Could you check a few things on this model? Use its own coordinates, in mm. A direction names the side the tool comes from. Give positions to 0.01 mm unless a question says otherwise; leave off trailing zeros. Write each loop counter-clockwise with the first axis right and the second up, starting at its lowest first coordinate (ties: lowest second). Pieces come first, ordered by that corner, then holes. Notation, with made-up numbers: (39, 68.5) -> (93, 68.5) arc R12 ccw to (93, 91.5) -> close; hole circle Ø1 at (-3, 14). An arc over 180 degrees is marked (long way). Write item = value, one per line. Start each with the question number.
```python
from build123d import *

# Parameters (mm, degrees)
ESQUISSE1_W                = 48
ESQUISSE1_H                = 24
EXTRUSION1_DEPTH           = 7.5
CONG_2_R                   = 5
CONG_5_R                   = 1
CONG_6_R                   = 1
ESQUISSE4_W                = 0.5
ESQUISSE4_H                = 18.982849842
EXTRUSION2_DEPTH           = 0.5
ESQUISSE5_R                = 0.25
EXTRUSION3_DEPTH           = 0.5
CHANFREIN1_SIZE            = 1
ESQUISSE6_R                = 1.5
EXTRUSION6_DEPTH           = 0.5
EXTRUSION6_DRAFT           = -45
EXTRUSION6_PROFILE_2_DEPTH = 0.5
EXTRUSION6_PROFILE_2_DRAFT = -45
EXTRUSION6_PROFILE_3_DEPTH = 0.5
EXTRUSION6_PROFILE_3_DRAFT = -45
EXTRUSION6_PROFILE_4_DEPTH = 0.5
EXTRUSION6_PROFILE_4_DRAFT = -45
EXTRUSION6_PROFILE_5_DEPTH = 0.5
EXTRUSION6_PROFILE_5_DRAFT = -45
EXTRUSION6_PROFILE_6_DEPTH = 0.5
EXTRUSION6_PROFILE_6_DRAFT = -45
EXTRUSION6_PROFILE_7_DEPTH = 0.5
EXTRUSION6_PROFILE_7_DRAFT = -45
EXTRUSION6_PROFILE_8_DEPTH = 0.5
EXTRUSION6_PROFILE_8_DRAFT = -45
EXTRUSION6_PROFILE_9_DEPTH = 0.5
EXTRUSION6_PROFILE_9_DRAFT = -45


with BuildPart() as part:
    # Esquisse1 → Extrusion1 (new body)
    with BuildSketch(Plane(origin=(0, 0, 0), x_dir=(1, 0, 0), z_dir=(0, 1, 0))):
        with Locations((24, 12)):
            Rectangle(ESQUISSE1_W, ESQUISSE1_H)
    extrude(amount=EXTRUSION1_DEPTH)

    # Congé2
    cong_2_edges = [part.edges().sort_by_distance(p)[0] for p in [
        (0, 3.75, -24),
        (48, 3.75, -24),
        (48, 3.75, 0),
        (0, 3.75, 0),
    ]]
    fillet(cong_2_edges, radius=CONG_2_R)

    # Congé5
    cong_5_edges = [part.edges().sort_by_distance(p)[0] for p in [
        (48, 7.5, -12),
        (24, 7.5, 0),
        (0, 7.5, -12),
        (24, 7.5, -24),
        (1.464466094, 7.5, -22.535533906),
        (1.464466094, 7.5, -1.464466094),
        (46.535533906, 7.5, -22.535533906),
        (46.535533906, 7.5, -1.464466094),
    ]]
    fillet(cong_5_edges, radius=CONG_5_R)

    # Congé6
    cong_6_edges = [part.edges().sort_by_distance(p)[0] for p in [
        (48, 0, -12),
        (0, 0, -12),
        (24, 0, -24),
        (24, 0, 0),
        (1.464466094, 0, -22.535533906),
        (1.464466094, 0, -1.464466094),
        (46.535533906, 0, -22.535533906),
        (46.535533906, 0, -1.464466094),
    ]]
    fillet(cong_6_edges, radius=CONG_6_R)

    # Esquisse4 → Extrusion2 (cut)
    with BuildSketch(Plane(origin=(0, 7.5, 0), x_dir=(1, 0, 0), z_dir=(0, 1, 0))):
        with Locations((24, 12)):
            Rectangle(ESQUISSE4_W, ESQUISSE4_H)
    extrude(amount=-EXTRUSION2_DEPTH, mode=Mode.SUBTRACT)

    # Esquisse5 → Extrusion3 (cut)
    with BuildSketch(Plane(origin=(0, 7.5, 0), x_dir=(1, 0, 0), z_dir=(0, 1, 0))):
        with Locations((24, 21.491424921)):
            Circle(ESQUISSE5_R)
        with Locations((24, 2.508575079)):
            Circle(ESQUISSE5_R)
    extrude(amount=-EXTRUSION3_DEPTH, mode=Mode.SUBTRACT)

    # Chanfrein1
    # the kernel refuses this chamfer: 1 mm, written as the material it takes off along each edge
    with BuildSketch(Plane(origin=(24, 7.5, -21.491424921), x_dir=(1, 0, 0), z_dir=(0, 0, 1))) as chanfrein1_piece_1_section:
        Polygon((0.25 + CHANFREIN1_SIZE, 0), (0.25, -CHANFREIN1_SIZE), (0.25, 0), align=None)
    chanfrein1_piece_1 = revolve(axis=Axis((24, 7.5, -21.491424921), (0, 1, 0)), revolution_arc=180, mode=Mode.PRIVATE)
    chanfrein1_piece_1 = split(chanfrein1_piece_1, bisect_by=Plane(origin=(24, 7, -21.964580549), z_dir=(0, 1, 0)), keep=Keep.TOP, mode=Mode.PRIVATE)
    add(chanfrein1_piece_1, mode=Mode.SUBTRACT)
    with BuildSketch(Plane(origin=(24.25, 7.5, -21.491424921), x_dir=(0.9996219169112968, 0.02749587661058651, 0), z_dir=(0, 0, 1))) as chanfrein1_piece_2_section:
        Polygon((CHANFREIN1_SIZE * 0.999621916911, -CHANFREIN1_SIZE * 0.0274958766106), (-CHANFREIN1_SIZE * 0.0274958766106, -CHANFREIN1_SIZE * 0.999621916911), (0, 0), align=None)
    chanfrein1_piece_2 = extrude(amount=18.982849842, mode=Mode.PRIVATE)
    chanfrein1_piece_2 = split(chanfrein1_piece_2, bisect_by=Plane(origin=(24.643401084, 7, -12), z_dir=(0, 1, 0)), keep=Keep.TOP, mode=Mode.PRIVATE)
    add(chanfrein1_piece_2, mode=Mode.SUBTRACT)
    with BuildSketch(Plane(origin=(24, 7.5, -2.508575079), x_dir=(-1, 0, 0), z_dir=(0, 0, -1))) as chanfrein1_piece_3_section:
        Polygon((0.25 + CHANFREIN1_SIZE, 0), (0.25, -CHANFREIN1_SIZE), (0.25, 0), align=None)
    chanfrein1_piece_3 = revolve(axis=Axis((24, 7.5, -2.508575079), (0, 1, 0)), revolution_arc=180, mode=Mode.PRIVATE)
    chanfrein1_piece_3 = split(chanfrein1_piece_3, bisect_by=Plane(origin=(24, 7, -2.035419451), z_dir=(0, 1, 0)), keep=Keep.TOP, mode=Mode.PRIVATE)
    add(chanfrein1_piece_3, mode=Mode.SUBTRACT)
    with BuildSketch(Plane(origin=(23.75, 7.5, -2.508575079), x_dir=(-0.9996219169112968, 0.02749587661058651, 0), z_dir=(0, 0, -1))) as chanfrein1_piece_4_section:
        Polygon((CHANFREIN1_SIZE * 0.999621916911, -CHANFREIN1_SIZE * 0.0274958766106), (-CHANFREIN1_SIZE * 0.0274958766106, -CHANFREIN1_SIZE * 0.999621916911), (0, 0), align=None)
    chanfrein1_piece_4 = extrude(amount=18.982849842, mode=Mode.PRIVATE)
    chanfrein1_piece_4 = split(chanfrein1_piece_4, bisect_by=Plane(origin=(23.356598916, 7, -12), z_dir=(0, 1, 0)), keep=Keep.TOP, mode=Mode.PRIVATE)
    add(chanfrein1_piece_4, mode=Mode.SUBTRACT)


with BuildPart() as extrusion6_tool:
    # Esquisse6 → Extrusion6 (with draft: the straight prism first)
    with BuildSketch(Plane(origin=(0, 7.5, 0), x_dir=(1, 0, 0), z_dir=(0, 1, 0))):
        with Locations((42, 6)):
            Circle(ESQUISSE6_R)
    extrude(amount=-EXTRUSION6_DEPTH)
    # Extrusion6: the draft: its side faces are tilted about the plane it starts from
    extrusion6_sides = [extrusion6_tool.faces().sort_by_distance(p)[0] for p in [
        (40.5, 7.25, -6),
    ]]
    draft(extrusion6_sides, Plane(origin=(0, 7.5, 0), x_dir=(1, 0, 0), z_dir=(0, 1, 0)), EXTRUSION6_DRAFT)


with BuildPart() as part_1:
    add(part.part)

    # Extrusion6: cut by extrusion6_tool
    add(extrusion6_tool.part, mode=Mode.SUBTRACT)


with BuildPart() as extrusion6_profile_2_tool:
    # Esquisse6 → Extrusion6 profile 2 (with draft: the straight prism first)
    with BuildSketch(Plane(origin=(0, 7.5, 0), x_dir=(1, 0, 0), z_dir=(0, 1, 0))):
        with Locations((30.25, 18)):
            Circle(ESQUISSE6_R)
    extrude(amount=-EXTRUSION6_PROFILE_2_DEPTH)
    # Extrusion6 profile 2: the draft: its side faces are tilted about the plane it starts from
    extrusion6_profile_2_sides = [extrusion6_profile_2_tool.faces().sort_by_distance(p)[0] for p in [
        (28.75, 7.25, -18),
    ]]
    draft(extrusion6_profile_2_sides, Plane(origin=(0, 7.5, 0), x_dir=(1, 0, 0), z_dir=(0, 1, 0)), EXTRUSION6_PROFILE_2_DRAFT)


with BuildPart() as part_2:
    add(part_1.part)

    # Extrusion6 profile 2: cut by extrusion6_profile_2_tool
    add(extrusion6_profile_2_tool.part, mode=Mode.SUBTRACT)


with BuildPart() as extrusion6_profile_3_tool:
    # Esquisse6 → Extrusion6 profile 3 (with draft: the straight prism first)
    with BuildSketch(Plane(origin=(0, 7.5, 0), x_dir=(1, 0, 0), z_dir=(0, 1, 0))):
        with Locations((11.875, 17)):
            Circle(ESQUISSE6_R)
    extrude(amount=-EXTRUSION6_PROFILE_3_DEPTH)
    # Extrusion6 profile 3: the draft: its side faces are tilted about the plane it starts from
    extrusion6_profile_3_sides = [extrusion6_profile_3_tool.faces().sort_by_distance(p)[0] for p in [
        (10.375, 7.25, -17),
    ]]
    draft(extrusion6_profile_3_sides, Plane(origin=(0, 7.5, 0), x_dir=(1, 0, 0), z_dir=(0, 1, 0)), EXTRUSION6_PROFILE_3_DRAFT)


with BuildPart() as part_3:
    add(part_2.part)

    # Extrusion6 profile 3: cut by extrusion6_profile_3_tool
    add(extrusion6_profile_3_tool.part, mode=Mode.SUBTRACT)


with BuildPart() as extrusion6_profile_4_tool:
    # Esquisse6 → Extrusion6 profile 4 (with draft: the straight prism first)
    with BuildSketch(Plane(origin=(0, 7.5, 0), x_dir=(1, 0, 0), z_dir=(0, 1, 0))):
        with Locations((17.75, 17)):
            Circle(ESQUISSE6_R)
    extrude(amount=-EXTRUSION6_PROFILE_4_DEPTH)
    # Extrusion6 profile 4: the draft: its side faces are tilted about the plane it starts from
    extrusion6_profile_4_sides = [extrusion6_profile_4_tool.faces().sort_by_distance(p)[0] for p in [
        (16.25, 7.25, -17),
    ]]
    draft(extrusion6_profile_4_sides, Plane(origin=(0, 7.5, 0), x_dir=(1, 0, 0), z_dir=(0, 1, 0)), EXTRUSION6_PROFILE_4_DRAFT)


with BuildPart() as part_4:
    add(part_3.part)

    # Extrusion6 profile 4: cut by extrusion6_profile_4_tool
    add(extrusion6_profile_4_tool.part, mode=Mode.SUBTRACT)


with BuildPart() as extrusion6_profile_5_tool:
    # Esquisse6 → Extrusion6 profile 5 (with draft: the straight prism first)
    with BuildSketch(Plane(origin=(0, 7.5, 0), x_dir=(1, 0, 0), z_dir=(0, 1, 0))):
        with Locations((6, 17)):
            Circle(ESQUISSE6_R)
    extrude(amount=-EXTRUSION6_PROFILE_5_DEPTH)
    # Extrusion6 profile 5: the draft: its side faces are tilted about the plane it starts from
    extrusion6_profile_5_sides = [extrusion6_profile_5_tool.faces().sort_by_distance(p)[0] for p in [
        (4.5, 7.25, -17),
    ]]
    draft(extrusion6_profile_5_sides, Plane(origin=(0, 7.5, 0), x_dir=(1, 0, 0), z_dir=(0, 1, 0)), EXTRUSION6_PROFILE_5_DRAFT)


with BuildPart() as part_5:
    add(part_4.part)

    # Extrusion6 profile 5: cut by extrusion6_profile_5_tool
    add(extrusion6_profile_5_tool.part, mode=Mode.SUBTRACT)


with BuildPart() as extrusion6_profile_6_tool:
    # Esquisse6 → Extrusion6 profile 6 (with draft: the straight prism first)
    with BuildSketch(Plane(origin=(0, 7.5, 0), x_dir=(1, 0, 0), z_dir=(0, 1, 0))):
        with Locations((11.875, 7)):
            Circle(ESQUISSE6_R)
    extrude(amount=-EXTRUSION6_PROFILE_6_DEPTH)
    # Extrusion6 profile 6: the draft: its side faces are tilted about the plane it starts from
    extrusion6_profile_6_sides = [extrusion6_profile_6_tool.faces().sort_by_distance(p)[0] for p in [
        (10.375, 7.25, -7),
    ]]
    draft(extrusion6_profile_6_sides, Plane(origin=(0, 7.5, 0), x_dir=(1, 0, 0), z_dir=(0, 1, 0)), EXTRUSION6_PROFILE_6_DRAFT)


with BuildPart() as part_6:
    add(part_5.part)

    # Extrusion6 profile 6: cut by extrusion6_profile_6_tool
    add(extrusion6_profile_6_tool.part, mode=Mode.SUBTRACT)


with BuildPart() as extrusion6_profile_7_tool:
    # Esquisse6 → Extrusion6 profile 7 (with draft: the straight prism first)
    with BuildSketch(Plane(origin=(0, 7.5, 0), x_dir=(1, 0, 0), z_dir=(0, 1, 0))):
        with Locations((6, 7)):
            Circle(ESQUISSE6_R)
    extrude(amount=-EXTRUSION6_PROFILE_7_DEPTH)
    # Extrusion6 profile 7: the draft: its side faces are tilted about the plane it starts from
    extrusion6_profile_7_sides = [extrusion6_profile_7_tool.faces().sort_by_distance(p)[0] for p in [
        (4.5, 7.25, -7),
    ]]
    draft(extrusion6_profile_7_sides, Plane(origin=(0, 7.5, 0), x_dir=(1, 0, 0), z_dir=(0, 1, 0)), EXTRUSION6_PROFILE_7_DRAFT)


with BuildPart() as part_7:
    add(part_6.part)

    # Extrusion6 profile 7: cut by extrusion6_profile_7_tool
    add(extrusion6_profile_7_tool.part, mode=Mode.SUBTRACT)


with BuildPart() as extrusion6_profile_8_tool:
    # Esquisse6 → Extrusion6 profile 8 (with draft: the straight prism first)
    with BuildSketch(Plane(origin=(0, 7.5, 0), x_dir=(1, 0, 0), z_dir=(0, 1, 0))):
        with Locations((17.75, 7)):
            Circle(ESQUISSE6_R)
    extrude(amount=-EXTRUSION6_PROFILE_8_DEPTH)
    # Extrusion6 profile 8: the draft: its side faces are tilted about the plane it starts from
    extrusion6_profile_8_sides = [extrusion6_profile_8_tool.faces().sort_by_distance(p)[0] for p in [
        (16.25, 7.25, -7),
    ]]
    draft(extrusion6_profile_8_sides, Plane(origin=(0, 7.5, 0), x_dir=(1, 0, 0), z_dir=(0, 1, 0)), EXTRUSION6_PROFILE_8_DRAFT)


with BuildPart() as part_8:
    add(part_7.part)

    # Extrusion6 profile 8: cut by extrusion6_profile_8_tool
    add(extrusion6_profile_8_tool.part, mode=Mode.SUBTRACT)


with BuildPart() as extrusion6_profile_9_tool:
    # Esquisse6 → Extrusion6 profile 9 (with draft: the straight prism first)
    with BuildSketch(Plane(origin=(0, 7.5, 0), x_dir=(1, 0, 0), z_dir=(0, 1, 0))):
        with Locations((36.125, 12)):
            Circle(ESQUISSE6_R)
    extrude(amount=-EXTRUSION6_PROFILE_9_DEPTH)
    # Extrusion6 profile 9: the draft: its side faces are tilted about the plane it starts from
    extrusion6_profile_9_sides = [extrusion6_profile_9_tool.faces().sort_by_distance(p)[0] for p in [
        (34.625, 7.25, -12),
    ]]
    draft(extrusion6_profile_9_sides, Plane(origin=(0, 7.5, 0), x_dir=(1, 0, 0), z_dir=(0, 1, 0)), EXTRUSION6_PROFILE_9_DRAFT)


with BuildPart() as part_9:
    add(part_8.part)

    # Extrusion6 profile 9: cut by extrusion6_profile_9_tool
    add(extrusion6_profile_9_tool.part, mode=Mode.SUBTRACT)


solid = part_9.part
```
(1) I'm going to push flat-ended pins straight in: pin 1 (1.5 mm diameter, centred on y = 5.5, z = -3.5, fed in from -X); pin 2 (0.6 mm diameter, centred on x = 12, z = -16.5, fed in from +Y). Where does each tip first touch, or does it pass through?
(2) On a 3-axis mill with a long thin cutter (end or side, diameter ignored), from which of +Z, -Z, +X, -X, +Y, -Y can I reach the whole of each face in a straight line? I mean faces 5 (the cylindrical face through (1, 4, -2)), 6 (the flat face through (6, 7, -7)). Say none if no direction works.
(3) Imagine slicing it at C-C (x = 24). Please give me the cut outline in (y, z).
(4) If I drill on line 1 along X through (y, z) = (7.25, -18.5); line 2 along X through (y, z) = (7.25, -15.25); line 3 along Z through (x, y) = (39.5, 7), over which ranges is the centre line in solid material (lowest first)? Write a range as from..to.
(5) Imagine slicing it at B-B (x = 17.75). Please give me the cut outline in (y, z).
(6) We'd pull the mould along Z, two halves only. Please class faces 1 (the cylindrical face through (0.301, 0.285, -11.902)), 2 (the conical face through (23.98, 7.14, -1.62)), 3 (the cylindrical face through (1, 4, -22)), 4 (the flat face through (18, 7, -17)): released by +Z, released by -Z, zero draft, split by the parting line, or undercut.
(7) Imagine slicing it at A-A (y = 5). Please give me the cut outline in (x, z).
Answers below:
q1.pin_1 = 0.06
q1.pin_2 = 7
q2.face_5 = +Z, -X, +Y, -Y
q2.face_6 = +Y
q3.outline = (0, -23) arc R1 ccw to (1, -24) -> (6.5, -24) arc R1 ccw to (7.5, -23) -> (7.5, -22.74) -> (7, -22.24) -> (7, -1.76) -> (7.5, -1.26) -> (7.5, -1) arc R1 ccw to (6.5, 0) -> (1, 0) arc R1 ccw to (0, -1) -> close
q4.line_1 = 0.34..23, 25..29.1, 31.4..47.66
q4.line_2 = 0.34..23, 25..47.66
q4.line_3 = -23.87..-0.13
q5.outline = (0, -23) arc R1 ccw to (1, -24) -> (6.5, -24) arc R1 ccw to (7.5, -23) -> (7.5, -18.5) -> (7, -18) -> (7, -16) -> (7.5, -15.5) -> (7.5, -8.5) -> (7, -8) -> (7, -6) -> (7.5, -5.5) -> (7.5, -1) arc R1 ccw to (6.5, 0) -> (1, 0) arc R1 ccw to (0, -1) -> close
q6.face_1 = zero draft
q6.face_2 = undercut
q6.face_3 = released by -Z
q6.face_4 = undercut
q7.outline = (0, -19) arc R5 ccw to (5, -24) -> (43, -24) arc R5 ccw to (48, -19) -> (48, -5) arc R5 ccw to (43, 0) -> (5, 0) arc R5 ccw to (0, -5) -> close
